Autodesk Inventor part; units mm, degrees
ref_plane "YZ Plane" through (0, 0, 0) normal (1, 0, 0) x (0, 1, 0)
ref_plane "XZ Plane" through (0, 0, 0) normal (0, 1, 0) x (-1, 0, 0)
ref_plane "XY Plane" through (0, 0, 0) normal (0, 0, 1) x (1, 0, 0)
sketch "Sketch1" plane through (0, 0, 0) normal (1, 0, 0) x (0, 1, 0)
  circle A0 centre (5.9226, 5.0314) radius 9.525
  line L0 (5.9226, 5.0314) -> (12.2726, 5.0314) construction
  line L1 (12.2726, 1.3724) -> (5.9287, -2.2974)
  line L2 (5.9287, -2.2974) -> (-0.4213, 1.3617)
  line L3 (-0.4213, 1.3617) -> (-0.4274, 8.6905)
  line L4 (-0.4274, 8.6905) -> (5.9164, 12.3602)
  line L5 (5.9164, 12.3602) -> (12.2664, 8.7012)
  line L6 (12.2664, 8.7012) -> (12.2726, 1.3724)
  point P0 (0, 0)
  dimension "d0" = 19.05
extrude "Extrusion1" add sketch "Sketch1" along normal blind 4.7244
properties part number "3D Model Spacer"
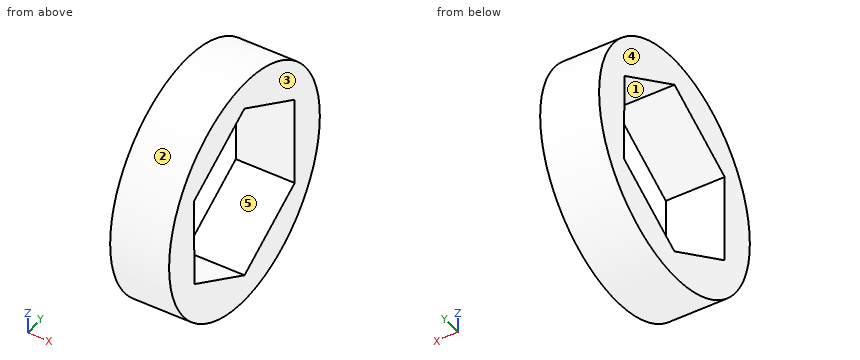
Check sheet for the modelled part. Datum: model origin and axes. Units: mm. Face numbers are marked on the shaded views. A direction names the side the tool comes from. Round coordinates to 2 decimals unless told otherwise and drop trailing zeros. Write each loop counter-clockwise with the first axis right and the second up, starting at its lowest first coordinate (ties: lowest second). Pieces come first, ordered by that corner, then holes. Notation, with made-up numbers: (2, 75.5) -> (61, 75.5) arc R28 cw to (61, 110.5) -> close; hole circle Ø4 at (87, 67.5). An arc over 180 degrees is marked (long way). Answer as CSV lines item,"result". Start each with the question number.
1) Go/stop test with a flat-tipped pin: P1, Ø1.5, axis at x = 1.5, y = -1, coming from the +Z side. Record where the tip stops, or that it passes through.
2) Section check B-B on y = 9.25. Enter the section's corners in (x, z).
3) Release check for a two-part mould opening along Y. For the marked faces 1, 2 and 3 record: pulls with the +Y half, pulls with the -Y half, needs draft (parallel to the pull), parting line crosses it, or undercut.
4) Section check D-D on y = -1.5. Enter the section's corners in (x, z), and give its area (3 significant figures).
5) Tool access check on the marked faces 4 and 5. Record the directions out of +Z, -Z, +X, -X, +Y, -Y that give a thin tool (end or side, any length) a straight path to the whole face; none if there is none.
6) Material ranges on line 1 (Y direction, x = 2.85, z = 7); line 2 (Y direction, x = 0.5, z = -2); line 3 (Z direction, x = 0.5, y = 4.25), recorded low to high. Write a range as from..to.
7) Section check A-A on z = 6.25. Enter the section's corners in (x, y).
Found:
1,P1,"stops at z = 12.29"
2,outline,"(0, -3.89) -> (4.72, -3.89) -> (4.72, -0.38) -> (0, -0.38) -> close; (0, 10.44) -> (4.72, 10.44) -> (4.72, 13.96) -> (0, 13.96) -> close"
3,face 1,"undercut"
3,face 2,"parting line crosses it"
3,face 3,"needs draft"
4,outline,"(0, -0.94) -> (4.72, -0.94) -> (4.72, 11) -> (0, 11) -> close"
4,area,"56.4 mm^2"
5,face 4,"+Z, -Z, -X, +Y, -Y"
5,face 5,"+X, -X"
6,line 1,"y = -3.4..-0.43, 12.27..15.24"
6,line 2,"y = -0.5..5.41, 6.44..12.35"
6,line 3,"z = -4.35..-1.33, 11.4..14.41"
7,outline,"(0, -3.52) -> (4.72, -3.52) -> (4.72, -0.43) -> (0, -0.43) -> close; (0, 12.27) -> (4.72, 12.27) -> (4.72, 15.37) -> (0, 15.37) -> close"
